Design review of the part built by this model. Coordinates are the model's own, in mm. A direction names the side the tool comes from. Coordinates: 2 decimals unless noted, no trailing zeros. Write each loop counter-clockwise with the first axis right and the second up, starting at its lowest first coordinate (ties: lowest second). Pieces come first, ordered by that corner, then holes. Notation, with made-up numbers: M 87.5,-17.75 L 127.5,-17.75 A11 cw 127.5,-0.75 Z; hole C 75.25,11 d7. An arc over 180 degrees is marked long. Write item = value, one per line.
Autodesk Inventor part; units mm, degrees
ref_plane "YZ Plane" through (0, 0, 0) normal (1, 0, 0) x (0, 1, 0)
ref_plane "XZ Plane" through (0, 0, 0) normal (0, 1, 0) x (-1, 0, 0)
ref_plane "XY Plane" through (0, 0, 0) normal (0, 0, 1) x (1, 0, 0)
sketch "Sketch1" plane through (0, 0, 0) normal (0, 0, 1) x (1, 0, 0)
  line L0 (0, 0) -> (300, 0)
  line L1 (300, 0) -> (300, 400)
  line L2 (300, 400) -> (0, 400)
  line L3 (0, 400) -> (0, 0)
  dimension "d0" = 300
  dimension "d1" = 400
extrude "Extrusion1" add sketch "Sketch1" along normal blind 90
sketch "Sketch2" plane through (0, 0, 90) normal (0, 0, 1) x (1, 0, 0)
  circle A0 centre (150, 300) radius 50
  point P0 (0, 0)
  dimension "d4" = 100
  dimension "d5" = 150
  dimension "d6" = 300
extrude "Extrusion2" cut sketch "Sketch2" against normal blind 100
sketch "Sketch4" plane through (0, 400, 0) normal (0, 1, 0) x (1, 0, 0)
  line L0 (10, -80) -> (290, -80)
  line L1 (290, -80) -> (290, -10)
  line L2 (290, -10) -> (10, -10)
  line L3 (10, -10) -> (10, -80)
  line L4 (0, 0) -> (0, -90)
  dimension "d12" = 70
  dimension "d13" = 280
  dimension "d14" = 10
  dimension "d15" = 10
extrude "Extrusion4" cut sketch "Sketch4" against normal blind 200
sketch "Sketch5" plane through (0, 0, 90) normal (0, 0, 1) x (1, 0, 0)
  line L0 (0, 205) -> (300, 205)
  line L1 (300, 400) -> (0, 400)
  line L2 (0, 400) -> (0, 0)
  line L3 (300, 0) -> (300, 400)
  line L4 (0, 205) -> (0, 172)
  line L5 (0, 172) -> (300, 172)
  line L6 (300, 0) -> (300, 400)
  line L7 (300, 205) -> (300, 172)
  dimension "d18" = 195
  dimension "d19" = 33
extrude "Extrusion5" add sketch "Sketch5" along normal blind 200 contours L0 L3 L5 L2
sketch "Sketch6" plane through (0, 0, 0) normal (0, -1, 0) x (1, 0, 0)
  line L0 (300, 90) -> (0, 90)
  line L1 (0, 0) -> (300, 0)
  line L2 (300, 0) -> (300, 90)
  line L3 (300, 90) -> (0, 90)
  line L4 (0, 90) -> (0, 0)
extrude "Extrusion6" cut sketch "Sketch6" against normal blind 172
sketch "Sketch7" plane through (0, 205, 90) normal (0, 1, 0) x (1, 0, 0)
  circle A0 centre (20, -180) radius 3
  circle A1 centre (20, -20) radius 3
  circle A2 centre (280, -23) radius 3
  circle A3 centre (280, -180) radius 3
  line L0 (300, -200) -> (0, -200)
  line L1 (0, 0) -> (0, -200)
  line L2 (300, 0) -> (0, 0)
  line L3 (300, 0) -> (300, -200)
  point P0 (0, 90)
  dimension "d24" = 20
  dimension "d25" = 20
  dimension "d26" = 6
  dimension "d27" = 20
  dimension "d28" = 20
  dimension "d29" = 20
  dimension "d30" = 20
  dimension "d31" = 20
  dimension "d32" = 20
extrude "Extrusion7" cut sketch "Sketch7" against normal blind 50 contours A0 | A1 | A2 | A3
properties part number "Baseservo"
Q1. The part is to be moulded in two halves that separate along Y. For faces 1 (the flat face through (115, 262, 0)), 2 (the cylindrical face through (113.148, 333.792, 5.07)), 3 (the flat face through (148, 205, 189)), say which applies: +Y half, -Y half, draft (parallel to the pull), parting line (faces both ways), or undercut.
Check result:
face_1 = draft
face_2 = undercut
face_3 = +Y half
Q2. Consider section D-D, the plane x = 213. State the section outline as (y, z) points.
Check result:
outline = M 172,0 L 400,0 L 400,10 L 200,10 L 200,80 L 400,80 L 400,90 L 205,90 L 205,290 L 172,290 Z
Q3. Consider section C-C, the plane y = 243. State the section outline as (x, z) points.
Check result:
outline = M 0,0 L 300,0 L 300,90 L 0,90 Z; hole M 10,10 L 290,10 L 290,80 L 10,80 Z
Q4. Consider section A-A, the plane x = 150. State the section outline as (y, z) points.
Check result:
outline = M 172,0 L 250,0 L 250,10 L 200,10 L 200,80 L 250,80 L 250,90 L 205,90 L 205,290 L 172,290 Z; M 350,0 L 400,0 L 400,10 L 350,10 Z; M 350,80 L 400,80 L 400,90 L 350,90 Z
Q5. Machinability: for faces 4 (the flat face through (115, 347, 90)), 5 (the flat face through (117, 346, 80)), 6 (the flat face through (162, 400, 81)), which of the approach directions +Z, -Z, +X, -X, +Y, -Y give a long, thin tool a straight path to every point of the face, cutting with its end or side? Answer none if there is none.
Check result:
face_4 = +Z, +X, -X, +Y
face_5 = +Y
face_6 = +Z, -Z, +X, -X, +Y
Q6. Wall thickness on line 1 (Z direction, x = 20, y = 181.5); line 2 (X direction, y = 194, z = 270); line 3 (Z direction, x = 170, y = 250): over which ranges is each line inside the solid? List them lowest first.
Check result:
line_1 = 0 to 107, 113 to 267, 273 to 290
line_2 = 0 to 17, 23 to 277, 283 to 300
line_3 = 0 to 10, 80 to 90
Q7. For P1, Ø5, axis at x = 234, y = 216.5, coming from the +Z side; P2, Ø1, axis at x = 225.5, z = 167.5, coming from the +Y side, all flat-tipped, find the tip position at first contact; note any pin that passes through.
Check result:
P1 = 90
P2 = 205
Q8. Consider section B-B, the plane y = 300. State the section outline as (x, z) points, and give its area (3 significant figures).
Check result:
outline = M 0,0 L 100,0 L 100,10 L 10,10 L 10,80 L 100,80 L 100,90 L 0,90 Z; M 200,0 L 300,0 L 300,90 L 200,90 L 200,80 L 290,80 L 290,10 L 200,10 Z
area = 5,400 mm²
